Geometry: see drawing. Coordinates: mm, zero at the bounding-box minimum. A direction names the side the tool comes from. Coordinates: 2 decimals unless noted, no trailing zeros. Write each loop counter-clockwise with the first axis right and the second up, starting at its lowest first coordinate (ties: lowest second). Pieces come first, ordered by that corner, then holes. Notation, with made-up numbers: (36, -26.75) - (92, -26.75) arc R23 cw to (92, 4.25) - close; hole circle Ø9 at (9.25, 39). An arc over 180 degrees is marked (long way). Use CSV: the item, a comma, the result in double quotes.
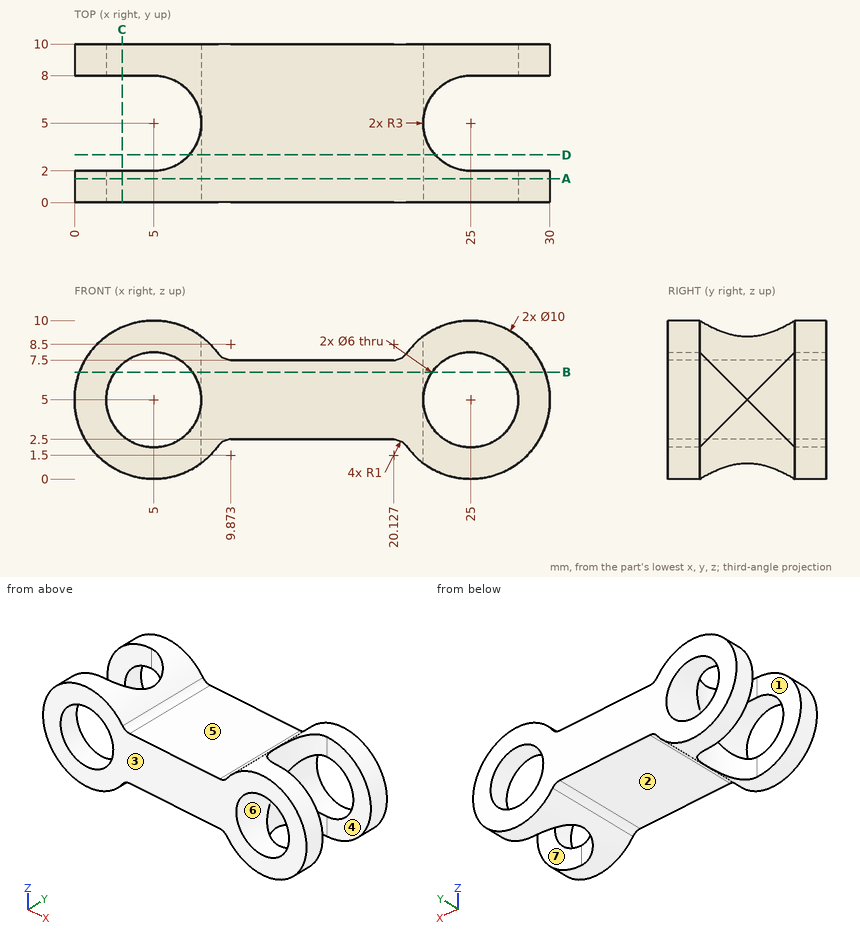
(1) Cut plane B-B on z = 6.75. Return loops of the section in (x, y).
Check values:
outline,"(0.32, 0) - (2.56, 0) - (2.56, 2) - (0.32, 2) - close; (0.32, 8) - (2.56, 8) - (2.56, 10) - (0.32, 10) - close; (7.44, 0) - (22.56, 0) - (22.56, 3.25) arc R3 cw to (22.56, 6.75) - (22.56, 10) - (7.44, 10) - (7.44, 6.75) arc R3 cw to (7.44, 3.25) - close; (27.44, 0) - (29.68, 0) - (29.68, 2) - (27.44, 2) - close; (27.44, 8) - (29.68, 8) - (29.68, 10) - (27.44, 10) - close"
(2) Reachability of the marked faces 1, 2, 3 and 4 from +Z, -Z, +X, -X, +Y, -Y: full face, straight path, thin tool, end or side. Return the list, or none.
Check values:
face 1,"+Z, -Z, -X"
face 2,"-Z, +Y, -Y"
face 3,"+Z, -Z, +X, -X, -Y"
face 4,"+Z, -Z, +X"
(3) Cut plane C-C on x = 3. Return loops of the section in (y, z).
Check values:
outline,"(0, 0.42) - (2, 0.42) - (2, 2.76) - (0, 2.76) - close; (0, 7.24) - (2, 7.24) - (2, 9.58) - (0, 9.58) - close; (8, 0.42) - (10, 0.42) - (10, 2.76) - (8, 2.76) - close; (8, 7.24) - (10, 7.24) - (10, 9.58) - (8, 9.58) - close"
(4) Cut plane A-A on y = 1.5. Return loops of the section in (x, z), and give its area (3 significant figures).
Check values:
outline,"(9.06, 2.08) arc R1 cw to (9.87, 2.5) - (20.13, 2.5) arc R1 cw to (20.94, 2.08) arc R5 ccw (long way) to (20.94, 7.92) arc R1 cw to (20.13, 7.5) - (9.87, 7.5) arc R1 cw to (9.06, 7.92) arc R5 ccw (long way) to start; hole circle Ø6 at (5, 5); hole circle Ø6 at (25, 5)"
area,"153 mm^2"
(5) Cut plane D-D on y = 3. Return loops of the section in (x, z).
Check values:
outline,"(7.24, 0.53) arc R5 ccw to (9.06, 2.08) arc R1 cw to (9.87, 2.5) - (20.13, 2.5) arc R1 cw to (20.94, 2.08) arc R5 ccw to (22.76, 0.53) - (22.76, 3) arc R3 cw to (22.76, 7) - (22.76, 9.47) arc R5 ccw to (20.94, 7.92) arc R1 cw to (20.13, 7.5) - (9.87, 7.5) arc R1 cw to (9.06, 7.92) arc R5 ccw to (7.24, 9.47) - (7.24, 7) arc R3 cw to (7.24, 3) - close"
(6) Draft query along Z for the marked faces 5, 6 and 7. Return one class per face: pulls with the +Z half, pulls with the -Z half, needs draft (parallel to the pull), parting line crosses it, or undercut.
Check values:
face 5,"pulls with the +Z half"
face 6,"undercut"
face 7,"needs draft"
(7) Pin query (flat end, axial travel): pin 1 Ø1 at (x, y) = (8, 4) entering from +Z; pin 2 Ø5 at (y, z) = (4, 3) entering from -X (1 decimal); pin 3 Ø1 at (x, y) = (21, 8.5) entering from +Z; pin 4 Ø3.5 at (x, z) = (25, 5) entering from +Y. Return the tip coordinate at first contact, or that it passes through.
Check values:
pin 1,"z = 9.23"
pin 2,"x = 0"
pin 3,"z = 8.57"
pin 4,"through"
(8) Ray query, probe 1 along Y at (x, z) = (26.5, 2); probe 2 along X at (y, z) = (8.75, 6.25); probe 3 along Z at (x, y) = (19.5, 7.5). Return the intervals inside material, ascending. Write a range as from..to.
Check values:
probe 1,"0..2, 8..10"
probe 2,"0.16..2.27, 7.73..22.27, 27.73..29.84"
probe 3,"2.5..7.5"
